Autodesk Inventor part; units mm, degrees
ref_plane "YZ Plane" through (0, 0, 0) normal (1, 0, 0) x (0, 1, 0)
ref_plane "XZ Plane" through (0, 0, 0) normal (0, 1, 0) x (-1, 0, 0)
ref_plane "XY Plane" through (0, 0, 0) normal (0, 0, 1) x (1, 0, 0)
sketch "Sketch1" plane through (0, 0, 0) normal (0, 0, 1) x (1, 0, 0)
  line L0 (0, 0) -> (64, 0)
  line L1 (64, 20) -> (0, 20)
  line L2 (0, 20) -> (0, 0)
  arc A0 (89.7812, -4.7516) -> (89.7812, 24.7516) centre (92.5, 10) ccw
  line L3 (64, 20) -> (89.7812, 24.7516)
  line L4 (64, 0) -> (89.7812, -4.7516)
  circle A1 centre (92.5, 10) radius 1.5
  dimension "d5" = 30
  dimension "d6" = 92.5
  dimension "d9" = 3
  dimension "d26" = 20
extrude "Extrusion1" add sketch "Sketch1" along normal blind 3 contours L2 L1 L3 A0 L4 L0 | A1
extrude "Extrusion2" cut sketch "Sketch1" along normal blind 10 contours A1
sketch "Sketch3" plane through (0, 0, 3) normal (0, 0, 1) x (1, 0, 0)
  circle A0 centre (92.5, 10) radius 1.5
  circle A1 centre (92.5, 10) radius 1.5
  line L0 (92.5, 10) -> (128.0101, 10) construction
  arc A2 (96.8308, 16.1692) -> (98.6692, 14.3308) centre (97.75, 15.25) ccw
  arc A3 (100.5192, 16.1808) -> (98.6808, 18.0192) centre (99.6, 17.1) ccw
  line L1 (96.8308, 16.1692) -> (98.6808, 18.0192)
  line L2 (100.5192, 16.1808) -> (98.6692, 14.3308)
  point P0 (0, 0)
  dimension "d18" = 2.6
  dimension "d19" = 2.6
extrude "Extrusion3" cut sketch "Sketch3" against normal blind 10 contours L1 A3 L2 A2
pattern_circular "Circular Pattern1" count 4 over 360 about axis through (92.5, 10, 0) along (0, 0, 1) of "Extrusion3"
sketch "Sketch4" plane through (0, 0, 3) normal (0, 0, 1) x (1, 0, 0)
  circle A0 centre (5.625, 5) radius 1.6
  circle A1 centre (16.875, 15) radius 1.6
  point P0 (0, 0)
  dimension "d27" = 3.2
  dimension "d28" = 3.2
extrude "Extrusion4" cut sketch "Sketch4" against normal blind 10
sketch "Sketch5" plane through (0, 0, 3) normal (0, 0, 1) x (1, 0, 0)
  line L0 (91.1147, 10.2457) -> (94, 10)
  circle A0 centre (92.5, 10) radius 1.5
  circle A1 centre (16.875, 15) radius 1.6
  line L1 (17.5362, 16.511) -> (16.875, 15)
  circle A2 centre (5.625, 5) radius 1.6
  line L2 (16.875, 15) -> (5.625, 5)
  circle A3 centre (16.875, 15) radius 2.032
  circle A4 centre (5.625, 5) radius 2.032
  point P0 (0, 0)
  dimension "d31" = 4.064
  dimension "d32" = 4.064
extrude "Extrusion5" cut sketch "Sketch5" against normal blind 10 contours A1 L2 L1 | A3 | A2 | A4 | L1 L2 A1
sketch "Sketch6" plane through (0, 0, 3) normal (0, 0, 1) x (1, 0, 0)
  circle A0 centre (92.5, 10) radius 1.5
  line L0 (92.8215, 11.4329) -> (92.5, 10)
  circle A1 centre (92.5, 10) radius 3.0734
  point P0 (0, 0)
  dimension "d35" = 6.1468
extrude "Extrusion6" cut sketch "Sketch6" against normal blind 10
sketch "Sketch7" plane through (0, 0, 3) normal (0, 0, 1) x (1, 0, 0)
  point P0 (0, 0)
sketch "Sketch8" plane through (0, 0, 3) normal (0, 0, 1) x (1, 0, 0)
  point P0 (0, 0)
sketch "Sketch9" plane through (0, 0, 3) normal (0, 0, 1) x (1, 0, 0)
  point P0 (0, 0)
sketch "Sketch10" plane through (0, 0, 3) normal (0, 0, 1) x (1, 0, 0)
  line L0 (0, 0) -> (64, 0)
  line L1 (22.5, 0) -> (22.5, 20)
  line L2 (64, 20) -> (0, 20)
  line L3 (0, 20) -> (0, 0)
  line L4 (64, 20) -> (64, 0)
  dimension "d38" = 22.5
extrude "Extrusion7" add sketch "Sketch10" along normal blind 2 contours L1 L2 L4 L0
fillet "Fillet1" radius 2 1 edges at (64, 10, 5)
properties part number "Arm"
The model under review builds one solid part; all positions refer to its coordinate system, in mm. A direction names the side the tool comes from. Give positions to 0.01 mm unless a question says otherwise; leave off trailing zeros. Order: outer loops, then holes, each group sorted by start corner. A loop starts at its lowest first (then second) coordinate and runs counter-clockwise, first axis right, second up. Notation, with made-up numbers: M 66,75.5 L 115,75.5 A13 cw 115,90.5 Z; hole C -30.5,89.5 d9. An arc over 180 degrees is marked long. One line per question, with ' | ' between items. Start each with the question number.
1) Mouldability with a two-part tool opening along X and no side actions: class faces 1 (the face through (39, 0, 2)), 2 (the face through (100.5, 1.96, 1.52)), 3 (the face through (76.71, -2.343, 1.479)), 4 (the face through (87.23, 17.11, 1.52)) as pulls with the +X half, pulls with the -X half, needs draft (parallel to the pull), parting line crosses it, or undercut.
2) Clearance check with flat-ended pins moving along their axes: P1, Ø3, axis at x = 84, y = 0, coming from the +Z side; P2, Ø2, axis at y = 0.5, z = 1.5, coming from the +X side. State where each tip first meets the part, or that it passes through.
3) Consider section B-B, the plane z = 0.8. Give the boundary of the cut face in (x, y) (3 decimals).
4) Consider section D-D, the plane x = 75. Give the boundary of the cut face in (y, z), then the cut area to 3 significant figures.
5) Wall thickness on L1, parallel to Y at x = 92.5, z = 2.1; L2, parallel to X at y = 5, z = 1.4; L3, parallel to X at y = 15, z = 2.05: over which ranges is each line inside the solid? List them lowest first. Write a range as from..to.
6) Consider section A-A, the plane x = 92.5. Give the boundary of the cut face in (y, z), then the cut area to 3 significant figures.
7) For faces 5 (the face through (53, 10, 0)), 6 (the face through (99.61, 15.27, 1.52)), 7 (the face through (40, 20, 2)), 8 (the face through (85, 10, 3)), list the 3-axis set-ups (+Z, -Z, +X, -X, +Y, -Y) from which the entire face can be reached by the end or side of a thin tool; tool diameter is ignored.
8) Consider section C-C, the plane x = 36.5. Give the boundary of the cut face in (y, z).
Found:
1) face 1: needs draft | face 2: undercut | face 3: pulls with the -X half | face 4: undercut
2) P1: stops at z = 3 | P2: stops at x = 104.86
3) outline: M 0,0 L 64,0 L 89.781,-4.752 A15 ccw long 89.781,24.752 L 64,20 L 0,20 Z; hole C 5.625,5 d4.064; hole C 16.875,15 d4.064; hole M 84.481,3.819 A1.3 ccw 86.319,1.981 L 88.169,3.831 A1.3 ccw 86.331,5.669 Z; hole M 84.481,16.181 L 86.331,14.331 A1.3 ccw 88.169,16.169 L 86.319,18.019 A1.3 ccw Z; hole C 92.5,10 d6.147; hole M 96.831,3.831 L 98.681,1.981 A1.3 ccw 100.519,3.819 L 98.669,5.669 A1.3 ccw Z; hole M 96.831,16.169 A1.3 ccw 98.669,14.331 L 100.519,16.181 A1.3 ccw 98.681,18.019 Z
4) outline: M -2.03,0 L 22.03,0 L 22.03,3 L -2.03,3 Z | area: 72.2 mm²
5) L1: y = -5..6.93, 13.07..25 | L2: x = 0..3.59, 7.66..85.66, 88.53..96.47, 99.34..106.64 | L3: x = 0..14.84, 18.91..85.66, 88.53..96.47, 99.34..106.64
6) outline: M -5,0 L 6.93,0 L 6.93,3 L -5,3 Z; M 13.07,0 L 25,0 L 25,3 L 13.07,3 Z | area: 71.6 mm²
7) face 5: -Z, +X, -X, +Y, -Y | face 6: +Z, -Z | face 7: +Z, -Z, -X, +Y | face 8: +Z, +X, +Y, -Y
8) outline: M 0,0 L 20,0 L 20,5 L 0,5 Z
